from build123d import *

# Parameters (mm, degrees)
SKETCH1_R           = 1.6
SKETCH1_R_2         = 2
SKETCH1_R_3         = 1.65
SKETCH1_R_4         = 6
BOSS_EXTRUDE2_DEPTH = 1.5875
BOSS_EXTRUDE3_START = -1.5875
BOSS_EXTRUDE3_DEPTH = 1.5875
SKETCH4_R           = 4.4
SKETCH4_R_2         = 2.1
CUT_EXTRUDE1_DEPTH  = 1.5875


with BuildPart() as part:
    # Sketch1 → Boss-Extrude2 (new body)
    with BuildSketch(Plane(origin=(0, 0, 0), x_dir=(1, 0, 0), z_dir=(0, 1, 0))):
        with BuildLine():
            Line((57.785577921, -3.804263015), (46.607089569, 48.169037391))
            ThreePointArc((46.607089569, 48.169037391), (54.607089569, 56.169037391), (46.607089569, 64.169037391))
            Line((46.607089569, 64.169037391), (46.607089569, 96.669037391))
            ThreePointArc((46.607089569, 96.669037391), (9.774896481, 73.010639225), (15.974342375, 29.675928865))
            Line((15.974342375, 29.675928865), (13.412399058, 22.705365919))
            ThreePointArc((13.412399058, 22.705365919), (-1.253243965, 6.307648563), (13.412399058, -10.090068793))
            Line((13.412399058, -10.090068793), (44.33382846, -62.316035804))
            ThreePointArc((44.33382846, -62.316035804), (50, -75.963557391), (55.66617154, -62.316035804))
            Line((55.66617154, -62.316035804), (59.462816555, -19.578912916))
            ThreePointArc((59.462816555, -19.578912916), (67.394599283, -10.759075533), (57.785577921, -3.804263015))
        make_face()
        with Locations(Location((27.233234802, -19.578912916, 0), (0, 0, 270))):
            Circle(SKETCH1_R, mode=Mode.SUBTRACT)
        with Locations(Location((44.33382846, -37.488387538, 0), (0, 0, 270))):
            Circle(SKETCH1_R, mode=Mode.SUBTRACT)
        with Locations(Location((40.089632361, 12.439739227, 0), (0, 0, 270))):
            Circle(SKETCH1_R, mode=Mode.SUBTRACT)
        with Locations(Location((12.19812376, 17.202869591, 0), (0, 0, 270))):
            Circle(SKETCH1_R_2, mode=Mode.SUBTRACT)
        with Locations(Location((26.141977063, 9.356280839, 0), (0, 0, 270))):
            Circle(SKETCH1_R_3, mode=Mode.SUBTRACT)
        with Locations(Location((4.351535007, 3.259016288, 0), (0, 0, 270))):
            Circle(SKETCH1_R_2, mode=Mode.SUBTRACT)
        with Locations(Location((18.295388311, -4.587572465, 0), (0, 0, 270))):
            Circle(SKETCH1_R_3, mode=Mode.SUBTRACT)
        with Locations(Location((46.607089569, 56.169037391, 0), (0, 0, 270))):
            Circle(SKETCH1_R_4, mode=Mode.SUBTRACT)
        with Locations(Location((59.462816555, -11.60242182, 0), (0, 0, 270))):
            Circle(SKETCH1_R_4, mode=Mode.SUBTRACT)
        with Locations(Location((50, -67.963557391, 0), (0, 0, 270))):
            Circle(SKETCH1_R_4, mode=Mode.SUBTRACT)
    extrude(amount=BOSS_EXTRUDE2_DEPTH)

    # Sketch3 → Boss-Extrude3 (add)
    with BuildSketch(Plane(origin=(0, 1.5875, 0), x_dir=(1, 0, 0), z_dir=(0, 1, 0)).offset(BOSS_EXTRUDE3_START)):
        with BuildLine():
            ThreePointArc((56.343437375, 106.672616503), (38.029280092, 122.267991205), (25.551142047, 101.702968958))
            ThreePointArc((25.551142047, 101.702968958), (27.87263843, 97.242332074), (31.478334129, 93.737252132))
            ThreePointArc((31.478334129, 93.737252132), (38.901984022, 95.929336038), (46.607089569, 96.669037391))
            Line((46.607089569, 96.669037391), (46.607089569, 92.08436081))
            ThreePointArc((46.607089569, 92.08436081), (53.685796044, 97.903157102), (56.343437375, 106.672616503))
        make_face()
        with BuildLine():
            ThreePointArc((46.607089569, 96.669037391), (38.901984022, 95.929336038), (31.478334129, 93.737252132))
            ThreePointArc((31.478334129, 93.737252132), (38.83054718, 90.968883646), (46.607089569, 92.08436081))
            Line((46.607089569, 92.08436081), (46.607089569, 96.669037391))
        make_face()
        with BuildLine():
            Line((25.551142047, 101.702968958), (23.684957519, 89.558045497))
            ThreePointArc((23.684957519, 89.558045497), (27.467237121, 91.860997946), (31.478334129, 93.737252132))
            ThreePointArc((31.478334129, 93.737252132), (27.87263843, 97.242332074), (25.551142047, 101.702968958))
        make_face()
        with BuildLine():
            Line((14.718034312, 31.202296417), (13.412399058, 22.705365919))
            Line((13.412399058, 22.705365919), (15.974342375, 29.675928865))
            ThreePointArc((15.974342375, 29.675928865), (15.33687379, 30.431446107), (14.718034312, 31.202296417))
        make_face()
    extrude(amount=BOSS_EXTRUDE3_DEPTH)

    # Sketch4 → Cut-Extrude1 (cut)
    with BuildSketch(Plane(origin=(0, 1.5875, 0), x_dir=(1, 0, 0), z_dir=(0, 1, 0))):
        with Locations(Location((40.546257627, 106.672616503, 0), (0, 0, 270))):
            Circle(SKETCH4_R)
        with Locations(Location((40.546257627, 117.14024961, 0), (0, 0, 270))):
            Circle(SKETCH4_R_2)
        with Locations(Location((30.07862452, 106.672616503, 0), (0, 0, 270))):
            Circle(SKETCH4_R_2)
        with Locations(Location((51.013890734, 106.672616503, 0), (0, 0, 270))):
            Circle(SKETCH4_R_2)
        with Locations(Location((40.546257627, 96.204983396, 0), (0, 0, 270))):
            Circle(SKETCH4_R_2)
    extrude(amount=-CUT_EXTRUDE1_DEPTH, mode=Mode.SUBTRACT)


solid = part.part
Geometry: final body of the model. Coordinates: model frame, mm. Coordinates: 2 decimals unless noted, no trailing zeros. Loops run counter-clockwise (first coordinate to the right, second up) from the corner with the lowest first, then second, coordinate; pieces in that order, holes last. Notation, with made-up numbers: (34, 22.5) - (86, 22.5) arc R14 ccw to (86, 34.5) - close; hole circle Ø2 at (-37, 51.25). An arc over 180 degrees is marked (long way). One line per question, with ' | ' between items. Start each with the question number.
(1) First-contact query: pin 1 (7 mm diameter, centred on x = 46.61, z = -56.17, fed in from +Y); pin 2 (5.5 mm diameter, centred on x = 26.14, z = -9.36, fed in from +Y). Flat tips, straight axial feed; report the tip coordinate or a pass-through.
(2) Cut plane A-A on y = 0.55. Count the separate pieces of the cut face and the enclosed holes in it, and give its area (3 significant figures).
(3) Cut plane B-B on z = -26. Output: boundary loops of the cut face in (x, y), and give its area (3 significant figures).
(4) Ray query, L1, parallel to Z at x = 59.5, y = 1.15; L2, parallel to Z at x = 27.5, y = 0.4; L3, parallel to X at y = 0.8, z = -12. Return the intervals inside material, ascending. Write a range as from..to.
(5) Draft query along X for faces 1 (the cylindrical face through (6.65, 0.78, -62.78)), 2 (the cylindrical face through (49.74, 0.78, 75.96)), 3 (the cylindrical face through (46.871, 0.783, -62.163)). Return one class per face: +X half, -X half, draft (parallel to the pull), parting line (faces both ways), or undercut.
Here are the results:
1) pin 1: through | pin 2: y = 1.59
2) separate pieces: 1 | enclosed holes: 15 | area: 6,470 mm²
3) outline: (13.92, 0) - (51.38, 0) - (51.38, 1.59) - (13.92, 1.59) - close | area: 59.5 mm²
4) L1: 3.63..5.6, 17.6..19.58 | L2: -115.58..-10.29, -8.42..18, 21.16..33.88 | L3: -0.24..38.55, 41.63..54.39
5) face 1: -X half | face 2: parting line | face 3: undercut
